Could you check a few things on this model? Use its own coordinates, in mm. Face numbers are marked on the shaded views. A direction names the side the tool comes from. Coordinates: 2 decimals unless noted, no trailing zeros. Order: outer loops, then holes, each group sorted by start corner. A loop starts at its lowest first (then second) coordinate and runs counter-clockwise, first axis right, second up. Notation, with made-up numbers: (-24, -27) - (9, -27) arc R16 ccw to (9, -8) - close; hole circle Ø6 at (25.5, 76.5). An arc over 180 degrees is marked (long way). One line per item, written item: value.
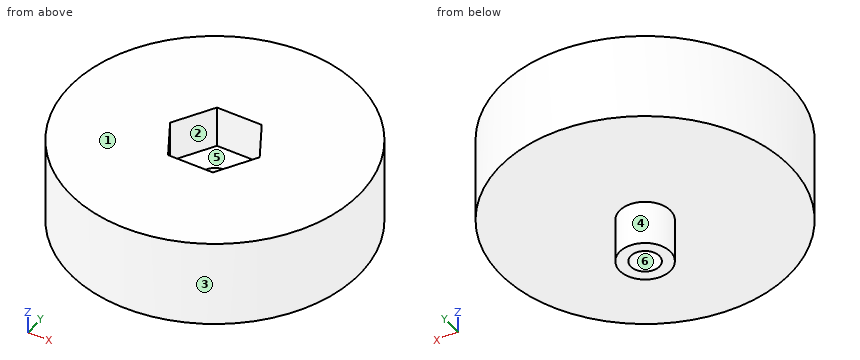
from build123d import *

# Parameters (mm, degrees)
SKETCH16_R           = 22.75
BOSS_EXTRUDE9_DEPTH  = 6.5
BOSS_EXTRUDE10_START = 7.1
SKETCH18_R           = 22.75
SKETCH18_R_2         = 2.25
BOSS_EXTRUDE10_DEPTH = 7.1
BOSS_EXTRUDE11_START = 7
SKETCH19_R           = 4
SKETCH19_R_2         = 2.25
BOSS_EXTRUDE11_DEPTH = 7


with BuildPart() as part:
    # Sketch16 → Boss-Extrude9 (new body)
    with BuildSketch(Plane.XY):
        with Locations(Location((0, 0, 0), (0, 0, 180))):
            Circle(SKETCH16_R)
        Polygon((7.101408311, 0), (3.550704156, 6.15), (-3.550704156, 6.15), (-7.101408311, 0), (-3.550704156, -6.15), (3.550704156, -6.15), align=None, mode=Mode.SUBTRACT)
    extrude(amount=BOSS_EXTRUDE9_DEPTH)

    # Sketch18 → Boss-Extrude10 (add)
    with BuildSketch(Plane(origin=(0, 0, 0), x_dir=(-1, 0, 0), z_dir=(0, 0, -1)).offset(BOSS_EXTRUDE10_START)):
        Circle(SKETCH18_R)
        Circle(SKETCH18_R_2, mode=Mode.SUBTRACT)
    extrude(amount=-BOSS_EXTRUDE10_DEPTH)

    # Sketch19 → Boss-Extrude11 (add)
    with BuildSketch(Plane(origin=(0, 0, -7.1), x_dir=(-1, 0, 0), z_dir=(0, 0, -1)).offset(BOSS_EXTRUDE11_START)):
        Circle(SKETCH19_R)
        Circle(SKETCH19_R_2, mode=Mode.SUBTRACT)
    extrude(amount=-BOSS_EXTRUDE11_DEPTH)


solid = part.part
Item 1: I'm going to push flat-ended pins straight in: pin 1 Ø3 at (x, z) = (-10.5, 1) entering from +Y; pin 2 Ø2 at (x, z) = (0, 3) entering from +Y; pin 3 Ø6 at (x, z) = (-3, -7) entering from -Y. Where does each tip first touch, or does it pass through?
Conclusion:
pin 1: y = 20.89
pin 2: y = 22.75
pin 3: y = -22.75
Item 2: I want a section at D-D on z = -3.75. Please give me the cut outline in (x, y).
Conclusion:
outline: circle Ø45.5 at (0, 0); hole circle Ø4.5 at (0, 0)
Item 3: If I drill on probe 1 along Y at (x, z) = (0, -5); probe 2 along Y at (x, z) = (0, -10.25); probe 3 along Z at (x, y) = (-13, 18.5), over which ranges is the centre line in solid material (lowest first)?
Conclusion:
probe 1: -22.75 to -2.25, 2.25 to 22.75
probe 2: -4 to -2.25, 2.25 to 4
probe 3: -7.1 to 6.5
Item 4: I want a section at C-C on y = 3. Please give me the cut outline in (x, z), then the cut area to 3 significant figures.
Conclusion:
outline: (-22.55, -7.1) - (-2.65, -7.1) - (-2.65, -14.1) - (2.65, -14.1) - (2.65, -7.1) - (22.55, -7.1) - (22.55, 6.5) - (5.37, 6.5) - (5.37, 0) - (-5.37, 0) - (-5.37, 6.5) - (-22.55, 6.5) - close
area: 581 mm²
Item 5: Thinking about a two-plate mould opening in Y: for the marked faces 1, 2 and 3, which applies, pulls with the +Y half, pulls with the -Y half, needs draft (parallel to the pull), parting line crosses it, or undercut?
Conclusion:
face 1: needs draft
face 2: undercut
face 3: parting line crosses it
Item 6: I want a section at A-A on z = 2.75. Please give me the cut outline in (x, y), then the cut area to 3 significant figures.
Conclusion:
outline: circle Ø45.5 at (0, 0); hole (-7.1, 0) - (-3.55, -6.15) - (3.55, -6.15) - (7.1, 0) - (3.55, 6.15) - (-3.55, 6.15) - close
area: 1,490 mm²
Item 7: I want a section at B-B on x = 0. Please give me the cut outline in (y, z), then the cut area to 3 significant figures.
Conclusion:
outline: (-22.75, -7.1) - (-4, -7.1) - (-4, -14.1) - (-2.25, -14.1) - (-2.25, 0) - (-6.15, 0) - (-6.15, 6.5) - (-22.75, 6.5) - close; (2.25, -14.1) - (4, -14.1) - (4, -7.1) - (22.75, -7.1) - (22.75, 6.5) - (6.15, 6.5) - (6.15, 0) - (2.25, 0) - close
area: 531 mm²
Item 8: For the marked faces 4, 5 and 6, which set-ups out of +Z, -Z, +X, -X, +Y, -Y let a thin tool reach every point of the face, with its end or its side?
Conclusion:
face 4: -Z
face 5: +Z
face 6: +Z, -Z
